from build123d import *

# Parameters (mm, degrees)
SKETCH1_R           = 5.5
SKETCH1_R_2         = 1.16205649
BOSS_EXTRUDE1_DEPTH = 4
FILLET1_R           = 5


with BuildPart() as part:
    # Sketch1 → Boss-Extrude1 (new body)
    with BuildSketch(Plane(origin=(0, 0, 0), x_dir=(1, 0, 0), z_dir=(0, 1, 0))):
        Polygon((-9.811758465, -5.619740701), (0.188241535, -8.249999209), (11.79974155, 0), (14, 7.8), (8.848495573, 9.5), (0.188241535, 9.5), (-9.811758465, 5), (-14, 0), align=None)
        Circle(SKETCH1_R, mode=Mode.SUBTRACT)
        with Locations((-10, 0)):
            Circle(SKETCH1_R_2, mode=Mode.SUBTRACT)
        with Locations((8.660254038, 5)):
            Circle(SKETCH1_R_2, mode=Mode.SUBTRACT)
    extrude(amount=BOSS_EXTRUDE1_DEPTH)

    # Fillet1
    fillet1_edges = [part.edges().sort_by_distance(p)[0] for p in [
        (-14, 2, 0),
        (0.188241535, 2, -9.5),
        (14, 2, -7.8),
        (0.188241535, 2, 8.249999209),
    ]]
    fillet(fillet1_edges, radius=FILLET1_R)


solid = part.part
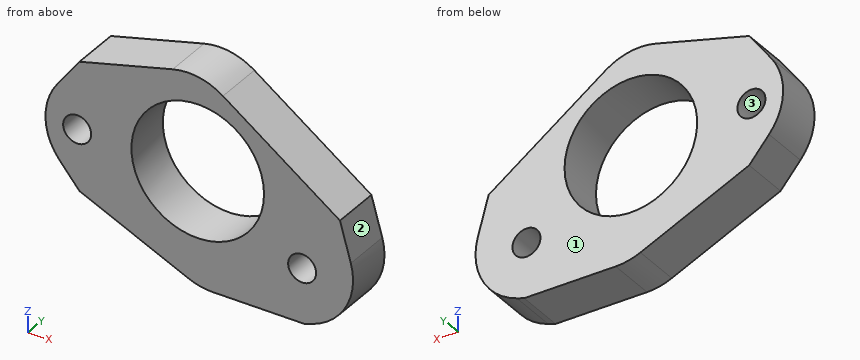
The model under review builds one solid part; all positions refer to its coordinate system, in mm. Face numbers are marked on the shaded views. Round coordinates to 2 decimals unless told otherwise and drop trailing zeros. Loops run counter-clockwise (first coordinate to the right, second up) from the corner with the lowest first, then second, coordinate; pieces in that order, holes last. Notation, with made-up numbers: (70.25, 22.5) -> (78.25, 22.5) arc R19 cw to (78.25, 52.5) -> close; hole circle Ø2 at (66.25, 71). An arc over 180 degrees is marked (long way). Answer as CSV lines item,"result".
1) Add section C-C on z = 0.5. Write out the cut boundary in (x, y).
Geometry results:
outline,"(-12.62, 0) -> (-11.05, 0) -> (-11.05, 4) -> (-12.62, 4) -> close; (-8.95, 0) -> (-5.48, 0) -> (-5.48, 4) -> (-8.95, 4) -> close; (5.48, 0) -> (11.1, 0) -> (11.1, 4) -> (5.48, 4) -> close"
2) Add section B-B on x = 0. Write out the cut boundary in (y, z).
Geometry results:
outline,"(0, -9.34) -> (4, -9.34) -> (4, -5.5) -> (0, -5.5) -> close; (0, 5.5) -> (4, 5.5) -> (4, 7.75) -> (0, 7.75) -> close"
3) For P1, Ø1.4, axis at x = -10, z = 0, coming from the -Y side; P2, Ø6, axis at x = -5.5, z = 4.5, coming from the -Y side, all flat-tipped, find the tip position at first contact; note any pin that passes through.
Geometry results:
P1,"passes through"
P2,"stops at y = 0"
4) Draft analysis for pull direction X (two halves, no side actions). For the marked faces 1, 2 and 3, state which applies: pulls with the +X half, pulls with the -X half, needs draft (parallel to the pull), parting line crosses it, or undercut.
Geometry results:
face 1,"needs draft"
face 2,"pulls with the +X half"
face 3,"undercut"
5) To check wall thickness, follow line 1 along X through (y, z) = (1, -0.5); line 2 along X through (y, z) = (3.45, 3.75); line 3 along Z through (x, y) = (-5, 2.85). State the ranges of each line that lie inside material, in increasing order. Write a range as from..to.
Geometry results:
line 1,"x = -12.58..-11.05, -8.95..-5.48, 5.48..11.94"
line 2,"x = -11.21..-4.02, 4.02..6.52"
line 3,"z = -7.17..-2.29, 2.29..6.89"
6) Add section A-A on y = 2.9. Write out the cut boundary in (x, z).
Geometry results:
outline,"(-11.64, 3.17) arc R5 ccw to (-11.46, -3.03) -> (-9.81, -5) -> (-0.79, -9.06) arc R5 ccw to (1.26, -9.5) -> (8.85, -9.5) -> (9.46, -9.3) arc R5 ccw to (12.7, -3.19) -> (11.8, 0) -> (2.09, 6.9) arc R5 ccw to (-2.07, 7.66) -> (-9.81, 5.62) -> close; hole circle Ø2.32 at (-10, 0); hole circle Ø11 at (0, 0); hole circle Ø2.32 at (8.66, -5)"
7) Add section D-D on x = -7. Write out the cut boundary in (y, z), plus the area to 3 significant figures.
Geometry results:
outline,"(0, -6.27) -> (4, -6.27) -> (4, 6.36) -> (0, 6.36) -> close"
area,"50.5 mm²"
